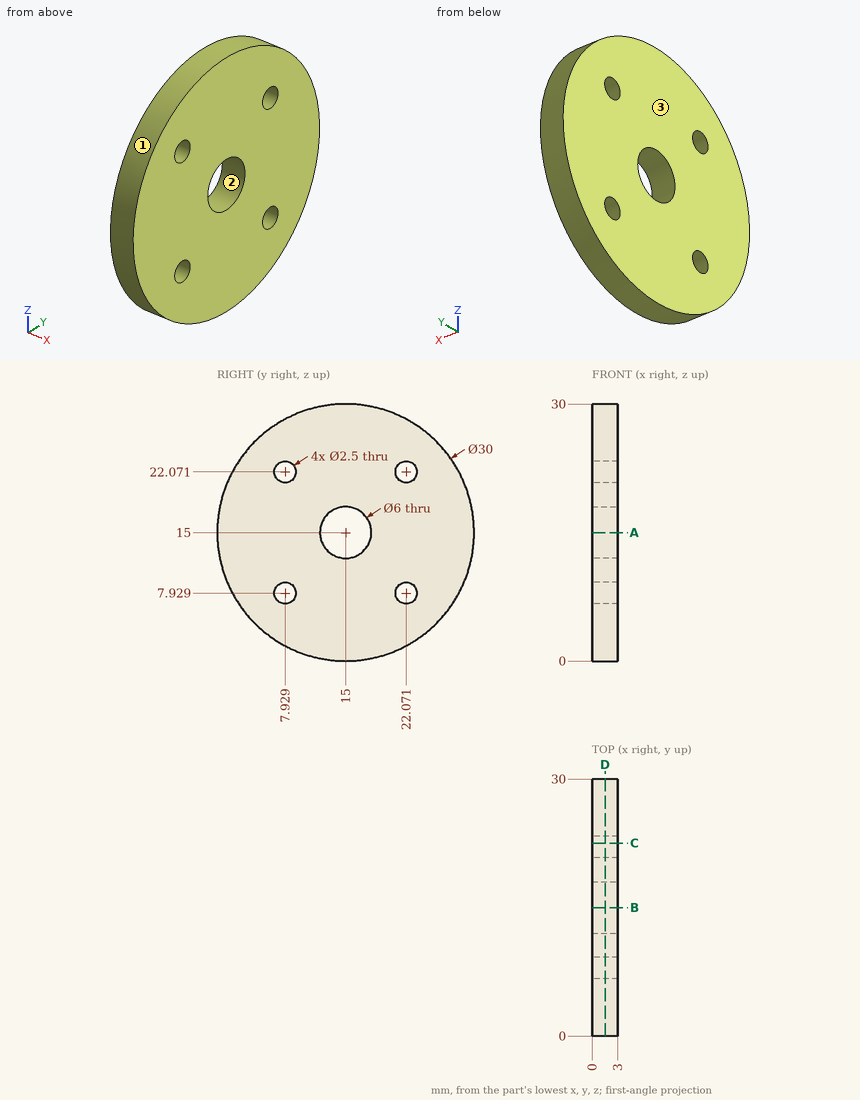
Study the drawing (mm; zero at the part's minimum x, y, z) and answer. Coordinates: 2 decimals unless noted, no trailing zeros. Loops run counter-clockwise (first coordinate to the right, second up) from the corner with the lowest first, then second, coordinate; pieces in that order, holes last. Notation, with made-up numbers: (8.25, -1.5) -> (38.25, -1.5) arc R26 ccw to (38.25, 26.5) -> close; hole circle Ø8 at (14, 9). An arc over 180 degrees is marked (long way). Answer in a Markdown table with one row per item. Add a question column.
1. Consider line 1 (Y direction, x = 2.9, z = 21.75); line 2 (Z direction, x = 2.8, y = 7.25); line 3 (Y direction, x = 1.2, z = 15). Determine where each line is inside the solid, lowest interval first. Write a range as [from, to].
2. The part is cut by section D-D, the plane x = 1.5. Write down the section's boundary in (y, z), then the cut area to 3 significant figures.
3. Determine the mould class of the marked faces 1, 2 and 3 for opening direction Z: +Z half, -Z half, draft (parallel to the pull), parting line (faces both ways), or undercut.
4. The part is cut by section C-C, the plane y = 22.5. Write down the section's boundary in (x, z).
5. Flat-ended cylindrical pins translate along their axes: P1, Ø1, axis at x = 0.5, y = 6, coming from the -Z side; P2, Ø5.5, axis at y = 15, z = 15, coming from the -X side. Find the tip coordinate at first contact, or state that the pin passes through.
6. The part is cut by section A-A, the plane z = 15. Write down the section's boundary in (x, y), then the cut area to 3 significant figures.
Answer below:
| question | item | result |
|---|---|---|
| 1 | line 1 | [1.6, 6.72], [9.14, 20.86], [23.28, 28.4] |
| 1 | line 2 | [2.16, 6.88], [8.98, 21.02], [23.12, 27.84] |
| 1 | line 3 | [0, 12], [18, 30] |
| 2 | outline | circle Ø30 at (15, 15); hole circle Ø2.5 at (7.93, 7.93); hole circle Ø2.5 at (7.93, 22.07); hole circle Ø6 at (15, 15); hole circle Ø2.5 at (22.07, 7.93); hole circle Ø2.5 at (22.07, 22.07) |
| 2 | area | 659 mm2 |
| 3 | face 1 | parting line |
| 3 | face 2 | undercut |
| 3 | face 3 | draft |
| 4 | outline | (0, 2.01) -> (3, 2.01) -> (3, 6.75) -> (0, 6.75) -> close; (0, 9.1) -> (3, 9.1) -> (3, 20.9) -> (0, 20.9) -> close; (0, 23.25) -> (3, 23.25) -> (3, 27.99) -> (0, 27.99) -> close |
| 5 | P1 | z = 2.64 |
| 5 | P2 | through |
| 6 | outline | (0, 0) -> (3, 0) -> (3, 12) -> (0, 12) -> close; (0, 18) -> (3, 18) -> (3, 30) -> (0, 30) -> close |
| 6 | area | 72.0 mm2 |
